Input: part model. Units: mm. Frame: model coordinates. A direction names the side the tool comes from. Give positions to 0.01 mm unless a question says otherwise; leave off trailing zeros. Write each loop counter-clockwise with the first axis right and the second up, starting at its lowest first coordinate (ties: lowest second). Pieces come first, ordered by that corner, then holes. Notation, with made-up numbers: (74, 48) -> (79, 48) arc R27 ccw to (79, 79) -> close; hole circle Ø3 at (-13.75, 73.5). An arc over 180 degrees is marked (long way). Return JSON: item names as keys, results as strings. Group by question number.
Item 1: Section B-B, the plane z = -4. Return loops of the section in (x, y), then the cut area to 3 significant figures.
Item 2: Pin query (flat end, axial travel): P1, Ø5, axis at x = -20, y = 11.5, coming from the +Z side; P2, Ø3, axis at x = -20.57, y = 11.88, coming from the +Z side; P3, Ø5, axis at x = 21.5, y = -12, coming from the +Z side; P4, Ø5.5, axis at x = 20.57, y = 11.88, coming from the -Z side. Return the tip coordinate at first contact, or that it passes through.
Item 3: Section D-D, the plane z = -8.5. Return loops of the section in (x, y), then the cut area to 3 significant figures.
Item 4: Mould query, pull axis Y, two halves, no side actions, for faces 3 (the face through (1, 2, -18)), 4 (the face through (-0.46, -20.23, 2.21)), 5 (the face through (-6.18, -27.82, 1.49)). Classes: released by +Y, released by -Y, zero draft, split by the parting line, or undercut.
Item 5: Section A-A, the plane y = 0. Return loops of the section in (x, z).
Item 6: Section C-C, the plane x = 0. Count the separate pieces of the cut face and the enclosed holes in it, then the cut area to 3 significant figures.
Item 7: Set-up query: faces 1 (the face through (-17.18, 12.94, 2.21)), 2 (the face through (0, -2, -16)). Return all of +Z, -Z, +X, -X, +Y, -Y with unobstructed straight access to the full face (end or side cutting, diameter ignored); none if empty.
Item 8: Line query: line 1 (Y direction, x = 0, z = 2.25); line 2 (Y direction, x = 0, z = -15.3); line 3 (Y direction, x = 0, z = 0.3). Output: solid intervals per line, ascending. Write a range as [from, to].
from build123d import *
from OCP.BRepFilletAPI import BRepFilletAPI_MakeChamfer

# Parameters (mm, degrees)
SKETCH1_R                      = 28.5
SKETCH1_R_2                    = 5.7
SKETCH1_R_3                    = 2
SKETCH1_R_4                    = 3
BOSS_EXTRUDE1_DEPTH            = 3
SKETCH2_R                      = 3.55
CUT_EXTRUDE1_DEPTH             = 2.4
BOSS_EXTRUDE2_START            = -12
SKETCH1_4_R                    = 5.7
SKETCH1_4_R_2                  = 3
BOSS_EXTRUDE2_DEPTH            = 12
BOSS_EXTRUDE3_START            = 6
SKETCH4_R                      = 5.7
SKETCH4_R_2                    = 2
BOSS_EXTRUDE3_DEPTH            = 6
CUT_EXTRUDE2_REACH             = 46.142
SKETCH3_R                      = 1.5
CUT_EXTRUDE2_DIRECTION_2_REACH = 46.142
FILLET1_R                      = 1
CHAMFER1_SIZE                  = 1.4
CHAMFER2_SIZE                  = 0.8
CHAMFER2_SIZE2                 = 1.385640646


with BuildPart() as part:
    # Sketch1 → Boss-Extrude1 (new body)
    # profile 1 of 2: a face of its own
    with BuildSketch(Plane(origin=(0, 0, 0), x_dir=(0, 1, 0), z_dir=(0, 0, 1))):
        with Locations(Location((0, 0, 0), (0, 0, 270))):
            Circle(SKETCH1_R)
        Circle(SKETCH1_R_2, mode=Mode.SUBTRACT)
        with Locations(Location((-23.75, 0, 0), (0, 0, 270))):
            Circle(SKETCH1_R_3, mode=Mode.SUBTRACT)
        with Locations(Location((-11.875, 20.56810334, 0), (0, 0, 270))):
            Circle(SKETCH1_R_3, mode=Mode.SUBTRACT)
        with Locations(Location((11.875, 20.56810334, 0), (0, 0, 270))):
            Circle(SKETCH1_R_3, mode=Mode.SUBTRACT)
        with Locations(Location((23.75, 0, 0), (0, 0, 270))):
            Circle(SKETCH1_R_3, mode=Mode.SUBTRACT)
        with Locations(Location((11.875, -20.56810334, 0), (0, 0, 270))):
            Circle(SKETCH1_R_3, mode=Mode.SUBTRACT)
        with Locations(Location((-11.875, -20.56810334, 0), (0, 0, 270))):
            Circle(SKETCH1_R_3, mode=Mode.SUBTRACT)
    # profile 2 of 2: a face of its own
    with BuildSketch(Plane(origin=(0, 0, 0), x_dir=(0, 1, 0), z_dir=(0, 0, 1))):
        Circle(SKETCH1_R_2)
        with Locations(Location((0, 0, 0), (0, 0, 270))):
            Circle(SKETCH1_R_4, mode=Mode.SUBTRACT)
    extrude(amount=BOSS_EXTRUDE1_DEPTH)

    # Sketch2 → Cut-Extrude1 (cut)
    with BuildSketch(Plane.XY.offset(3)):
        with Locations((-20.56810334, -11.875)):
            Circle(SKETCH2_R)
        with Locations((-20.56810334, 11.875)):
            Circle(SKETCH2_R)
        with Locations((0, 23.75)):
            Circle(SKETCH2_R)
        with Locations((20.56810334, 11.875)):
            Circle(SKETCH2_R)
        with Locations((20.56810334, -11.875)):
            Circle(SKETCH2_R)
        with Locations((0, -23.75)):
            Circle(SKETCH2_R)
    extrude(amount=-CUT_EXTRUDE1_DEPTH, mode=Mode.SUBTRACT)

    # Sketch1<4> → Boss-Extrude2 (add)
    with BuildSketch(Plane(origin=(0, 0, 0), x_dir=(0, 1, 0), z_dir=(0, 0, 1)).offset(BOSS_EXTRUDE2_START)):
        with Locations(Location((0, 0, 0), (0, 0, 270))):
            Circle(SKETCH1_4_R)
        with Locations(Location((0, 0, 0), (0, 0, 270))):
            Circle(SKETCH1_4_R_2, mode=Mode.SUBTRACT)
    extrude(amount=BOSS_EXTRUDE2_DEPTH)

    # Sketch4 → Boss-Extrude3 (add)
    with BuildSketch(Plane(origin=(0, 0, -12), x_dir=(1, 0, 0), z_dir=(0, 0, -1)).offset(BOSS_EXTRUDE3_START)):
        Circle(SKETCH4_R)
        with Locations(Location((0, 0, 0), (0, 0, 180))):
            Circle(SKETCH4_R_2, mode=Mode.SUBTRACT)
    extrude(amount=-BOSS_EXTRUDE3_DEPTH)

    # Sketch3 → Cut-Extrude2 (cut, up to next)
    with BuildSketch(Plane(origin=(0, 0, 0), x_dir=(-1, 0, 0), z_dir=(0, 1, 0)), mode=Mode.PRIVATE) as cut_extrude2_sk1:
        with Locations(Location((0, -4, 0), (0, 0, 90))):
            Circle(SKETCH3_R)
    cut_extrude2_tool1 = extrude(cut_extrude2_sk1.sketch, amount=-CUT_EXTRUDE2_REACH, mode=Mode.PRIVATE) & part.part
    add(cut_extrude2_tool1.solids().sort_by_distance((0, 0, -4))[0], mode=Mode.SUBTRACT)

    # Sketch3 → Cut-Extrude2 direction 2 (cut, up to next)
    with BuildSketch(Plane(origin=(0, 0, 0), x_dir=(-1, 0, 0), z_dir=(0, 1, 0)), mode=Mode.PRIVATE) as cut_extrude2_direction_2_sk1:
        with Locations(Location((0, -4, 0), (0, 0, 90))):
            Circle(SKETCH3_R)
    cut_extrude2_direction_2_tool1 = extrude(cut_extrude2_direction_2_sk1.sketch, amount=CUT_EXTRUDE2_DIRECTION_2_REACH, mode=Mode.PRIVATE) & part.part
    add(cut_extrude2_direction_2_tool1.solids().sort_by_distance((0, 0, -4))[0], mode=Mode.SUBTRACT)

    # Fillet1
    fillet1_edges = [part.edges().sort_by_distance(p)[0] for p in [
        (-28.5, 0, 0),
        (-28.5, 0, 3),
        (-5.7, 0, 0),
        (-5.7, 0, -18),
    ]]
    fillet(fillet1_edges, radius=FILLET1_R)

    # Chamfer1
    # the kernel refuses this chamfer: 1.4 mm, written as the material it takes off along each edge
    with BuildSketch(Plane(origin=(0, 0, -12), x_dir=(-1, 0, 0), z_dir=(0, -1, 0))) as chamfer1_piece_1_section:
        Polygon((2 + CHAMFER1_SIZE, 0), (2, CHAMFER1_SIZE), (2, 0), align=None)
    chamfer1_piece_1 = revolve(axis=Axis((0, 0, -12), (0, 0, -1)), mode=Mode.PRIVATE)
    chamfer1_piece_1 = chamfer1_piece_1 & Plane(origin=(0, 0, -12.902493822), x_dir=(1, 0, 0), z_dir=(0, 0, -1)) * Cylinder(3, 14, mode=Mode.PRIVATE)
    add(chamfer1_piece_1, mode=Mode.SUBTRACT)

    # Chamfer2: one chamfer whose edges measure the first distance from different faces: ONE call of the kernel's chamfer builder (chamfer() names one face for all edges)
    chamfer2_edges_1 = [part.edges().sort_by_distance(p)[0] for p in [
        (-3.55, -23.75, 0.6),
    ]]
    chamfer2_side_1 = [part.faces().sort_by_distance(p)[0] for p in [
        (-3.55, -23.75, 1.8),
    ]]
    chamfer2_edges_2 = [part.edges().sort_by_distance(p)[0] for p in [
        (17.01810334, -11.875, 0.6),
    ]]
    chamfer2_side_2 = [part.faces().sort_by_distance(p)[0] for p in [
        (17.01810334, -11.875, 1.8),
    ]]
    chamfer2_edges_3 = [part.edges().sort_by_distance(p)[0] for p in [
        (17.01810334, 11.875, 0.6),
    ]]
    chamfer2_side_3 = [part.faces().sort_by_distance(p)[0] for p in [
        (17.01810334, 11.875, 1.8),
    ]]
    chamfer2_edges_4 = [part.edges().sort_by_distance(p)[0] for p in [
        (-3.55, 23.75, 0.6),
    ]]
    chamfer2_side_4 = [part.faces().sort_by_distance(p)[0] for p in [
        (-3.55, 23.75, 1.8),
    ]]
    chamfer2_edges_5 = [part.edges().sort_by_distance(p)[0] for p in [
        (-24.11810334, 11.875, 0.6),
    ]]
    chamfer2_side_5 = [part.faces().sort_by_distance(p)[0] for p in [
        (-24.11810334, 11.875, 1.8),
    ]]
    chamfer2_edges_6 = [part.edges().sort_by_distance(p)[0] for p in [
        (-24.11810334, -11.875, 0.6),
    ]]
    chamfer2_side_6 = [part.faces().sort_by_distance(p)[0] for p in [
        (-24.11810334, -11.875, 1.8),
    ]]
    chamfer2 = BRepFilletAPI_MakeChamfer(part.part.solid().wrapped)
    for e in chamfer2_edges_1:
        chamfer2.Add(CHAMFER2_SIZE, CHAMFER2_SIZE2, e.wrapped, chamfer2_side_1[0].wrapped)  # the first distance lies on this face
    for e in chamfer2_edges_2:
        chamfer2.Add(CHAMFER2_SIZE, CHAMFER2_SIZE2, e.wrapped, chamfer2_side_2[0].wrapped)  # the first distance lies on this face
    for e in chamfer2_edges_3:
        chamfer2.Add(CHAMFER2_SIZE, CHAMFER2_SIZE2, e.wrapped, chamfer2_side_3[0].wrapped)  # the first distance lies on this face
    for e in chamfer2_edges_4:
        chamfer2.Add(CHAMFER2_SIZE, CHAMFER2_SIZE2, e.wrapped, chamfer2_side_4[0].wrapped)  # the first distance lies on this face
    for e in chamfer2_edges_5:
        chamfer2.Add(CHAMFER2_SIZE, CHAMFER2_SIZE2, e.wrapped, chamfer2_side_5[0].wrapped)  # the first distance lies on this face
    for e in chamfer2_edges_6:
        chamfer2.Add(CHAMFER2_SIZE, CHAMFER2_SIZE2, e.wrapped, chamfer2_side_6[0].wrapped)  # the first distance lies on this face
    add(Compound.cast(chamfer2.Shape()), mode=Mode.REPLACE)


solid = part.part
Answer below:
{
 "1": {"outline": "(-1.5, -5.5) -> (-1.5, -2.6) arc R3 cw to (-1.5, 2.6) -> (-1.5, 5.5) arc R5.7 ccw to start; (1.5, -5.5) arc R5.7 ccw to (1.5, 5.5) -> (1.5, 2.6) arc R3 cw to (1.5, -2.6) -> close", "area": "57.2 mm2"},
 "2": {"P1": "stops at z = 1.19", "P2": "passes through", "P3": "stops at z = 1.34", "P4": "stops at z = 0"},
 "3": {"outline": "circle Ø11.4 at (0, 0); hole circle Ø6 at (0, 0)", "area": "73.8 mm2"},
 "4": {"face 3": "zero draft", "face 4": "undercut", "face 5": "split by the parting line"},
 "5": {"outline": "(-28.5, 1) arc R1 ccw to (-27.5, 0) -> (-6.7, 0) arc R1 cw to (-5.7, -1) -> (-5.7, -17) arc R1 ccw to (-4.7, -18) -> (-2, -18) -> (-2, -13.4) -> (-3, -12.4) -> (-3, 3) -> (-27.5, 3) arc R1 ccw to (-28.5, 2) -> close; (2, -18) -> (4.7, -18) arc R1 ccw to (5.7, -17) -> (5.7, -1) arc R1 cw to (6.7, 0) -> (27.5, 0) arc R1 ccw to (28.5, 1) -> (28.5, 2) arc R1 ccw to (27.5, 3) -> (3, 3) -> (3, -12.4) -> (2, -13.4) -> close"},
 "6": {"separate pieces": "6", "enclosed holes": "0", "area": "207 mm2"},
 "7": {"face 1": "+Z", "face 2": "+Z, -Z"},
 "8": {"line 1": "y = [-28.47, -27.3], [-20.2, -3], [3, 20.2], [27.3, 28.47]", "line 2": "y = [-5.7, -2], [2, 5.7]", "line 3": "y = [-28.21, -25.75], [-21.75, -3], [3, 21.75], [25.75, 28.21]"}
}
